Read the model definition and answer for the solid it produces. Units are mm, in the model's axes. A direction names the side the tool comes from. Give positions to 0.01 mm unless a question says otherwise; leave off trailing zeros. Loops run counter-clockwise (first coordinate to the right, second up) from the corner with the lowest first, then second, coordinate; pieces in that order, holes last. Notation, with made-up numbers: (46, 7) - (69, 7) arc R29 ccw to (69, 39) - close; hole circle Ø9 at (34.25, 13). An arc over 180 degrees is marked (long way). Write item = value, one per line.
```python
from build123d import *

# Parameters (mm, degrees)
SKETCH_1_R      = 5
SKETCH_1_R_2    = 1.75
EXTRUDE_1_DEPTH = 10
EXTRUDE_START   = -10
EXTRUDE_2_DEPTH = 10
FILLET_1_R      = 10


with BuildPart() as part:
    # 草图1 → 凸台-拉伸1 (new body)
    # profile 1 of 3: a face of its own
    with BuildSketch(Plane(origin=(0, 0, 0), x_dir=(1, 0, 0), z_dir=(0, 1, 0))):
        Circle(SKETCH_1_R)
        with Locations(Location((0, 0, 0), (0, 0, 270))):
            Circle(SKETCH_1_R_2, mode=Mode.SUBTRACT)
    # profile 2 of 3: a face of its own
    with BuildSketch(Plane(origin=(0, 0, 0), x_dir=(1, 0, 0), z_dir=(0, 1, 0))):
        with BuildLine():
            Line((22, 5), (0, 5))
            ThreePointArc((0, 5), (3.535533906, 3.535533906), (5, 0))
            ThreePointArc((5, 0), (3.535533906, -3.535533906), (0, -5))
            Line((0, -5), (22, -5))
            ThreePointArc((22, -5), (17, 0), (22, 5))
        make_face()
    # profile 3 of 3: a face of its own
    with BuildSketch(Plane(origin=(0, 0, 0), x_dir=(1, 0, 0), z_dir=(0, 1, 0))):
        with Locations((22, 0)):
            Circle(SKETCH_1_R)
        with Locations(Location((22, 0, 0), (0, 0, 270))):
            Circle(SKETCH_1_R_2, mode=Mode.SUBTRACT)
    extrude(amount=EXTRUDE_1_DEPTH)

    # 草图2 → 凸台-拉伸2 (add)
    with BuildSketch(Plane(origin=(0, 10, 0), x_dir=(1, 0, 0), z_dir=(0, 1, 0)).offset(EXTRUDE_START)):
        with BuildLine():
            Line((22, -5), (25.0919928, -5))
            Line((25.0919928, -5), (41.259704507, 2.885519882))
            ThreePointArc((41.259704507, 2.885519882), (47.82742716, 5.211272452), (54.75, 6))
            Line((54.75, 6), (62.75, 6))
            Line((62.75, 6), (62.75, 12.87))
            Line((62.75, 12.87), (58.75, 12.87))
            ThreePointArc((58.75, 12.87), (34.552895834, 10.889316888), (11, 5))
            Line((11, 5), (22, 5))
            ThreePointArc((22, 5), (27, 0), (22, -5))
        make_face()
    extrude(amount=EXTRUDE_2_DEPTH)

    # 圆角1
    fillet_1_edges = [part.edges().sort_by_distance(p)[0] for p in [
        (11, 5, -5),
    ]]
    fillet(fillet_1_edges, radius=FILLET_1_R)


solid = part.part
```
1) Each of these flat-tipped pins is pushed along its axis until it touches: P1, Ø3, axis at x = 33.5, y = 2, coming from the -Z side; P2, Ø4, axis at x = 57.5, y = 4.5, coming from the +Z side; P3, Ø5, axis at x = 36, y = 8.5, coming from the -Z side. Where does it stop, or does it pass through?
Output:
P1 = -10.96
P2 = -6
P3 = -11.49
2) Find the intervals of material crossed by probe 1 along X at (y, z) = (4, 0); probe 2 along Z at (x, y) = (58.5, 5); probe 3 along Z at (x, y) = (3, 5.5), in increasing order.
Output:
probe_1 = -5 to -1.75, 1.75 to 20.25, 23.75 to 35.34
probe_2 = -12.87 to -6
probe_3 = -5 to 5
3) A cutting plane is placed at B-B on x = 22. Determine the outline of the cut face in (y, z).
Output:
outline = (0, -8.26) - (10, -8.26) - (10, -1.75) - (0, -1.75) - close; (0, 1.75) - (10, 1.75) - (10, 5) - (0, 5) - close
4) A cutting plane is placed at A-A on z = 0. Determine the outline of the cut face in (x, y), then the cut area to 3 significant figures.
Output:
outline = (-5, 0) - (-1.75, 0) - (-1.75, 10) - (-5, 10) - close; (1.75, 0) - (20.25, 0) - (20.25, 10) - (1.75, 10) - close; (23.75, 0) - (35.34, 0) - (35.34, 10) - (23.75, 10) - close
area = 333 mm²
5) The mould has two halves that part along X. Classify faces 4 (the face through (23.735, 4.93, -0.228)), 5 (the face through (35.652, 4.93, -11.066)), 6 (the face through (33.063, 4.93, 1.112)): pulls with the +X half, pulls with the -X half, needs draft (parallel to the pull), parting line crosses it, or undercut.
Output:
face_4 = undercut
face_5 = pulls with the -X half
face_6 = pulls with the +X half
6) A cutting plane is placed at C-C on y = 6.75. Determine the outline of the cut face in (x, z), then the cut area to 3 significant figures.
Output:
outline = (0, -5) - (9.38, -5) arc R10 cw to (12.49, -5.5) arc R148.79 ccw to (58.75, -12.87) - (62.75, -12.87) - (62.75, -6) - (54.75, -6) arc R30.77 cw to (41.26, -2.89) - (25.09, 5) - (0, 5) arc R5 ccw to start; hole circle Ø3.5 at (0, 0); hole circle Ø3.5 at (22, 0)
area = 645 mm²
7) A cutting plane is placed at D-D on z = -9.5. Determine the outline of the cut face in (x, y).
Output:
outline = (27.26, 0) - (62.75, 0) - (62.75, 10) - (27.26, 10) - close
8) A tool of negligible diameter and unlimited length cuts with its end or side. For faces 1 (the face through (59, 5, -6)), 2 (the face through (5, 5, -5)), 3 (the face through (28, 0, -4)), from which of +Z, -Z, +X, -X, +Y, -Y can it reach the whole face along a straight path? Write none if from no direction.
Output:
face_1 = +Z, +X, +Y, -Y
face_2 = -Z, -X, +Y, -Y
face_3 = +Z, -Z, +X, -X, -Y
